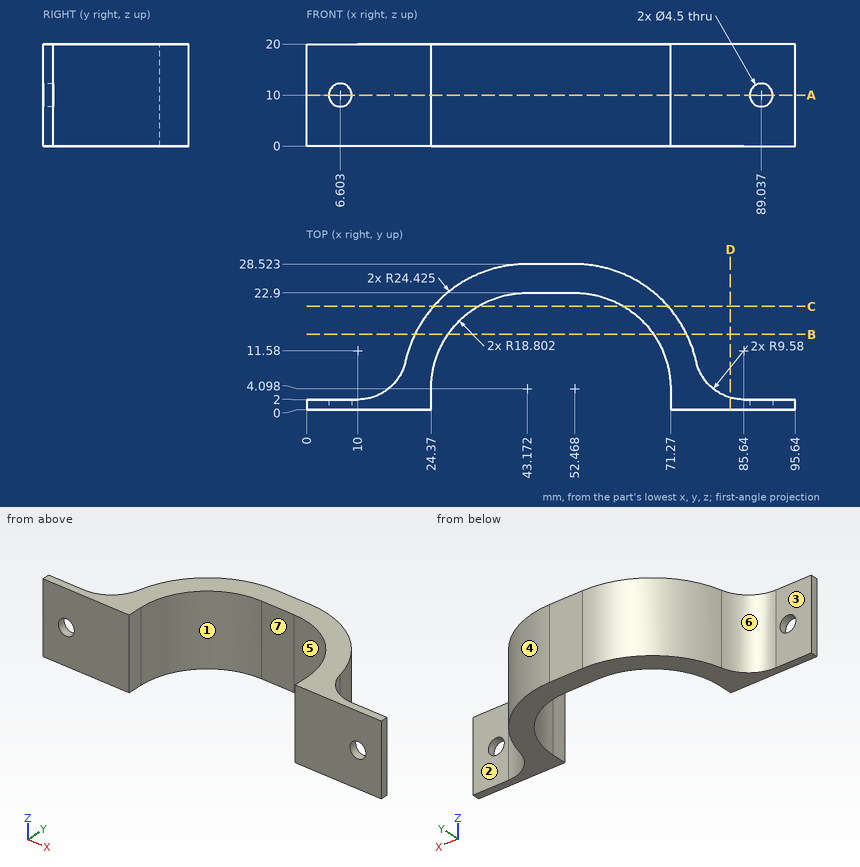
Can you work these out from the drawing? Everything is in mm from the part's minimum corner. A direction names the side the tool comes from. Coordinates: 2 decimals unless noted, no trailing zeros. Loops run counter-clockwise (first coordinate to the right, second up) from the corner with the lowest first, then second, coordinate; pieces in that order, holes last. Notation, with made-up numbers: (-37, 40.5) -> (17, 40.5) arc R18 cw to (17, 53.5) -> close; hole circle Ø2 at (-10, 26.5). An arc over 180 degrees is marked (long way). Return JSON: item names as keys, results as strings.
1) If we section it at A-A, the plane z = 10: Count the separate pieces of the cut face and the enclosed holes in it, then the cut area to 3 significant figures.
Results below:
{"separate pieces": "3", "enclosed holes": "0", "area": "566 mm²"}
2) If we section it at B-B, the plane y = 14.75: Write out the boundary of the cut face in (x, z).
Results below:
{"outline": "(21.19, 0) -> (27.68, 0) -> (27.68, 20) -> (21.19, 20) -> close; (67.96, 0) -> (74.45, 0) -> (74.45, 20) -> (67.96, 20) -> close"}
3) Thinking about a two-plate mould opening in X: for the marked faces 4, 5, 6 and 7, which applies, +X half, -X half, draft (parallel to the pull), parting line (faces both ways), or undercut?
Results below:
{"face 4": "+X half", "face 5": "undercut", "face 6": "-X half", "face 7": "undercut"}
4) If we section it at D-D, the plane x = 83: Write out the boundary of the cut face in (y, z).
Results below:
{"outline": "(0, 0) -> (2.37, 0) -> (2.37, 20) -> (0, 20) -> close"}
5) For the marked faces 1, 2 and 3, which set-ups out of +Z, -Z, +X, -X, +Y, -Y let a thin tool reach every point of the face, with its end or its side?
Results below:
{"face 1": "+Z, -Z, -Y", "face 2": "+Z, -Z, +X, +Y", "face 3": "+Z, -Z, -X, +Y"}
6) If we section it at C-C, the plane y = 20.25: Write out the boundary of the cut face in (x, z).
Results below:
{"outline": "(24.85, 0) -> (33.55, 0) -> (33.55, 20) -> (24.85, 20) -> close; (62.09, 0) -> (70.79, 0) -> (70.79, 20) -> (62.09, 20) -> close"}
7) I need wall thicknesses on line 1 (X direction, y = 16, z = 15.5) (1 decimal); line 2 (Y direction, x = 9.5, z = 11.5); line 3 (X direction, y = 11.25, z = 11.75) (1 decimal). Which ranges of each line are inside material? Lowest first, please. Write a range as from..to.
Results below:
{"line 1": "21.8..28.6, 67..73.8", "line 2": "0..2", "line 3": "19.8..25.8, 69.9..75.8"}
8) Will these pins go through, and if not, where does the flat tip stop? pin 1 (2 mm diameter, centred on y = 23.5, z = 13.5, fed in from +X); pin 2 (8 mm diameter, centred on x = 7, z = 14.5, fed in from +Y); pin 3 (5 mm diameter, centred on x = 65, z = 11.5, fed in from -Y); pin 4 (5 mm diameter, centred on x = 52.5, y = 19, fed in from +Z).
Results below:
{"pin 1": "x = 68.53", "pin 2": "y = 2.05", "pin 3": "y = 15.39", "pin 4": "through"}
